Read the model definition and answer for the solid it produces. Units are mm, in the model's axes. Give positions to 0.01 mm unless a question says otherwise; leave off trailing zeros. Order: outer loops, then holes, each group sorted by start corner. A loop starts at its lowest first (then second) coordinate and runs counter-clockwise, first axis right, second up. Notation, with made-up numbers: (-6.5, 82) - (29.5, 82) arc R14 ccw to (29.5, 100) - close; hole circle Ø8 at (69, 58). An arc over 180 degrees is marked (long way). Answer as CSV lines item,"result". Start each with the question number.
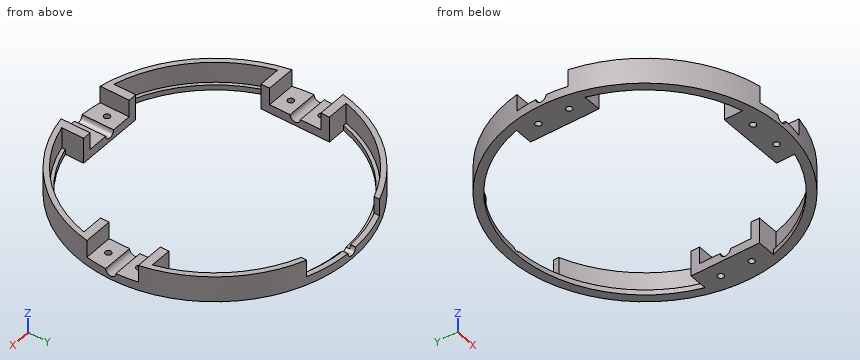
Autodesk Fusion 360 part; units mm, degrees
sketch "Sketch1" plane through (0, 0, 0) normal (0, 0, 1) x (1, 0, 0)
  circle A0 centre (0, 0) radius 80
  circle A1 centre (0, 0) radius 75
  line L0 (109.3577, 15) -> (-93.0881, 15) construction
  line L1 (20, 0) -> (2.5, 0)
  line L2 (109.3577, -15) -> (-93.0881, -15) construction
  line L3 (-78.5812, 15) -> (-61.5812, 15)
  line L4 (-78.5812, -15) -> (-61.5812, -15)
  line L5 (-97.5254, 20) -> (90.0497, 20) construction
  line L6 (-97.5254, -20) -> (90.0497, -20) construction
  line L7 (-77.4597, 20) -> (-61.5812, 20)
  line L8 (-77.4597, -20) -> (-61.5812, -20)
  line L9 (-61.5812, -15) -> (-61.5812, -20)
  line L10 (-61.5812, 15) -> (-61.5812, 20)
  line L11 (-20, -77.4597) -> (-20, -61.5812)
  line L12 (-15, -61.5812) -> (-20, -61.5812)
  line L13 (-15, -78.5812) -> (-15, -61.5812)
  line L14 (15, -78.5812) -> (15, -61.5812)
  line L15 (15, -61.5812) -> (20, -61.5812)
  line L16 (20, -77.4597) -> (20, -61.5812)
  line L17 (77.4597, -20) -> (61.5812, -20)
  line L18 (61.5812, -15) -> (61.5812, -20)
  line L19 (78.5812, -15) -> (61.5812, -15)
  line L20 (78.5812, 15) -> (61.5812, 15)
  line L21 (61.5812, 15) -> (61.5812, 20)
  line L22 (77.4597, 20) -> (61.5812, 20)
  line L23 (-28, 82.3691) -> (-28, 36.8916) construction
  line L24 (0, 2.5) -> (0, 20)
  line L25 (28, 82.3691) -> (28, 36.8916) construction
  line L26 (-33, 78.0405) -> (-33, 48.5416) construction
  line L27 (33, 78.0405) -> (33, 48.5416) construction
  line L28 (-28, 74.94) -> (-28, 69.5773)
  line L29 (28, 74.94) -> (28, 69.5773)
  line L30 (-61.5812, 15) -> (-61.5812, -15)
  line L31 (-15, -61.5812) -> (15, -61.5812)
  line L32 (61.5812, -15) -> (61.5812, 15)
  circle A2 centre (0, 0) radius 77
  dimension "d1" = 160
  dimension "d2" = -5
  dimension "d3" = 15
  dimension "d4" = 17
  dimension "d5" = 17
  dimension "d6" = 20
  dimension "d8" = 360
  dimension "d9" = 28
  dimension "d10" = 33
  dimension "d13" = -3
extrude "Extrude1" add sketch "Sketch1" along normal blind 15 contours A0 L20 L22 A2 | A0 L17 L19 A2 | A0 L22 L29 A2 | A1 L20 L22 A2 | A0 L16 L17 A2 | A1 L17 L19 A2 | A0 L28 L29 A2 | A1 L22 L29 A2 | A1 L20 L21 L22 | A0 L14 L16 A2 | A1 L16 L17 A2 | A1 L17 L18 L19 | A0 L7 L28 A2 | A1 L28 L29 A2 | A1 L14 L16 A2 | A0 L3 L7 A2 | A1 L7 L28 A2 | A0 L11 L13 A2 | A1 L14 L15 L16 | A1 L3 L7 A2 | A0 L8 L11 A2 | A1 L11 L13 A2 | A0 L4 L8 A2 | A1 L3 L7 L10 | A1 L8 L11 A2 | A1 L11 L12 L13 | A1 L4 L8 A2 | A1 L4 L8 L9 makes body 1 at (-69.1013, 40.3114, 10) makes body 2 at (18.8878, -77.7383, 5) makes body 3 at (-77.7383, -18.8878, 5)
extrude "Extrude2" add sketch "Sketch1" along normal blind 5 contours A0 L19 L20 A2 | A0 L20 L22 A2 | A0 L17 L19 A2 | A1 L19 L20 A2 | A1 L20 L22 A2 | A1 L17 L19 A2 | A1 L20 L21 L22 | A1 L19 L20 L32 | A0 L14 L16 A2 | A1 L17 L18 L19 | A0 L13 L14 A2 | A1 L14 L16 A2 | A0 L3 L7 A2 | A0 L11 L13 A2 | A1 L13 L14 A2 | A1 L14 L15 L16 | A0 L3 L4 A2 | A1 L3 L7 A2 | A1 L11 L13 A2 | A1 L13 L14 L31 | A0 L4 L8 A2 | A1 L3 L4 A2 | A1 L3 L7 L10 | A1 L11 L12 L13 | A1 L4 L8 A2 | A1 L3 L4 L30 | A1 L4 L8 L9 bodies 1 2 3
sketch "Sketch2" plane through (0, 0, 15) normal (0, 0, 1) x (-1, 0, 0)
  arc A0 (78.5812, 15) -> (15, 78.5812) centre (0, 0) ccw
  line L0 (15, 78.5812) -> (15, 61.5812)
  line L1 (15, 61.5812) -> (20, 61.5812)
  line L2 (20, 61.5812) -> (20, 72.2842)
  arc A1 (72.2842, 20) -> (20, 72.2842) centre (0, 0) ccw
  line L3 (72.2842, 20) -> (61.5812, 20)
  line L4 (61.5812, 20) -> (61.5812, 15)
  line L5 (61.5812, 15) -> (78.5812, 15)
  circle A2 centre (0, 0) radius 80
  circle A3 centre (0, 0) radius 77
  circle A4 centre (0, 0) radius 75
  line L6 (97.5254, 20) -> (-90.0497, 20)
  line L7 (97.5254, -20) -> (-90.0497, -20)
  line L8 (-20, 77.4597) -> (-20, 61.5812)
  line L9 (20, 77.4597) -> (20, 61.5812)
  line L10 (20, 72.2842) -> (20, 77.4597)
  line L11 (-20, 72.2842) -> (-20, 77.4597)
  line L12 (-72.2842, 20) -> (-77.4597, 20)
  line L13 (-72.2842, -20) -> (-77.4597, -20)
  line L14 (77.4597, 20) -> (72.2842, 20)
  line L15 (77.4597, -20) -> (72.2842, -20)
  dimension "d16" = -3
  dimension "d17" = -5
  dimension "d18" = 160
extrude "Extrude3" cut sketch "Sketch2" against normal blind 12 contours A1 A3 A4 L6 L9 L10 L14 | A3 A4 L7 L13 L15 | A3 A4 L6 L8 L11 L12 bodies 1
sketch "Sketch3" plane through (0, 0, 0) normal (0, 0, -1) x (1, 0, 0)
  arc A0 (-20, 72.2842) -> (-72.2842, 20) centre (0, 0) ccw
  line L0 (-20, 72.2842) -> (-20, 61.5812)
  line L1 (-20, 61.5812) -> (20, 61.5812)
  line L2 (20, 61.5812) -> (20, 72.2842)
  arc A1 (72.2842, 20) -> (20, 72.2842) centre (0, 0) ccw
  line L3 (72.2842, 20) -> (61.5812, 20)
  line L4 (61.5812, 20) -> (61.5812, -20)
  line L5 (61.5812, -20) -> (72.2842, -20)
  arc A2 (-72.2842, -20) -> (72.2842, -20) centre (0, 0) ccw
  line L6 (-72.2842, -20) -> (-61.5812, -20)
  line L7 (-61.5812, -20) -> (-61.5812, 20)
  line L8 (-61.5812, 20) -> (-72.2842, 20)
  circle A3 centre (0, 0) radius 70 construction
  line L9 (-17, 70) -> (15.5974, 70) construction
  circle A4 centre (9, 70) radius 1.75
  circle A5 centre (-9, 70) radius 1.75
  circle A6 centre (-70, 9) radius 1.75
  circle A7 centre (-70, -9) radius 1.75
  circle A8 centre (70, -9) radius 1.75
  circle A9 centre (70, 9) radius 1.75
  circle A10 centre (0, 0) radius 80
  dimension "d21" = 140
  dimension "d22" = 3.5
  dimension "d23" = 3.5
  dimension "d24" = 9
  dimension "d25" = 9
  dimension "d27" = 360
extrude "Extrude4" cut sketch "Sketch3" against normal blind 5 contours A4 | A5 | A6 | A7 | A8 | A9 bodies 1
sketch "Sketch4" plane through (0, 0, 15) normal (0, 0, 1) x (-1, 0, 0)
  line L0 (61.5812, -20) -> (74.3572, -20)
  arc A0 (-74.3572, -20) -> (74.3572, -20) centre (0, 0) ccw
  line L1 (-74.3572, -20) -> (-61.5812, -20)
  line L2 (-61.5812, -20) -> (-61.5812, -15)
  line L3 (-61.5812, -15) -> (-78.5812, -15)
  arc A1 (-78.5812, -15) -> (78.5812, -15) centre (0, 0) ccw
  line L4 (78.5812, -15) -> (61.5812, -15)
  line L5 (61.5812, -15) -> (61.5812, -20)
  line L6 (28, -82.3691) -> (28, -36.8916)
  line L7 (-28, -82.3691) -> (-28, -36.8916)
  circle A2 centre (0, 0) radius 75
  circle A3 centre (0, 0) radius 80
  line L8 (28, -74.94) -> (28, -69.5773)
  line L9 (-28, -74.94) -> (-28, -69.5773)
extrude "Extrude5" cut sketch "Sketch4" against normal blind 10 contours A0 L6 L7 A2 L8 L9 | A0 A1 L6 L7 A3 L8 L9 bodies 1
sketch "Sketch5" plane through (0, -61.5812, 0) normal (0, 1, 0) x (-1, 0, 0)
  line L0 (-15, 5) -> (-15, 15)
  line L1 (-15, 15) -> (-20, 15)
  line L2 (-20, 15) -> (-20, 0)
  line L3 (-20, 0) -> (20, 0)
  line L4 (20, 0) -> (20, 15)
  line L5 (20, 15) -> (15, 15)
  line L6 (15, 15) -> (15, 5)
  line L7 (15, 5) -> (-15, 5)
  circle A0 centre (0, 5) radius 3
  dimension "d32" = 6
extrude "Extrude6" cut sketch "Sketch5" against normal blind 18.419 contours L7 A0 picked at (-0.7219, 4.1708) bodies 1
pattern_circular "C-Pattern1" count 4 over 360 about axis through (0, 0, 1.75) along (0, 0, 1) of "Extrude6"
(1) Section B-B, the plane x = -42 is taken. Write down the section's boundary in (y, z), and give its area (3 significant figures).
(2) Section C-C, the plane z = 12 is taken. Write down the section's boundary in (x, y), and give its area (3 significant figures).
(3) Flat-ended cylindrical pins translate along their axes: pin 1 Ø4.5 at (x, y) = (70, 9) entering from +Z; pin 2 Ø5 at (y, z) = (30, 8.5) entering from -X; pin 3 Ø4 at (x, z) = (-70, 8.5) entering from -Y. Find the tip coordinate at first contact, or state that the pin passes through.
(4) Straight lines are drawn through the part: line 1 (X direction, y = -9, z = 3.25); line 2 (Y direction, x = -70, z = 3.5); line 3 (Y direction, x = -3, z = 0.75). For each, find the intervals that lie inside material, in ascending order. Write a range as [from, to].
(5) Section A-A, the plane y = 56 is taken. Write down the section's boundary in (x, z).
Checks:
1,outline,"(-68.09, 0) - (-62.14, 0) - (-62.14, 3) - (-64.54, 3) - (-64.54, 15) - (-68.09, 15) - close; (62.14, 0) - (68.09, 0) - (68.09, 15) - (64.54, 15) - (64.54, 3) - (62.14, 3) - close"
1,area,"121 mm²"
2,outline,"(-78.58, -15) arc R80 ccw to (-15, -78.58) - (-15, -61.58) - (-20, -61.58) - (-20, -74.36) arc R77 cw to (-74.36, -20) - (-61.58, -20) - (-61.58, -15) - close; (-78.58, 15) - (-61.58, 15) - (-61.58, 20) - (-74.36, 20) arc R77 cw to (-28, 71.73) - (-28, 74.94) arc R80 ccw to start; (15, -78.58) arc R80 ccw to (78.58, -15) - (61.58, -15) - (61.58, -20) - (74.36, -20) arc R77 cw to (20, -74.36) - (20, -61.58) - (15, -61.58) - close; (28, 71.73) arc R77 cw to (74.36, 20) - (61.58, 20) - (61.58, 15) - (78.58, 15) arc R80 ccw to (28, 74.94) - close"
2,area,"1,440 mm²"
3,pin 1,"stops at z = 5"
3,pin 2,"stops at x = -75.12"
3,pin 3,"stops at y = -42.14"
4,line 1,"x = [-79.49, -71.75], [-68.25, -61.58], [61.58, 68.25], [71.75, 79.49]"
4,line 2,"y = [-38.73, -32.08], [-20, -10.75], [-7.25, -2.6], [2.6, 7.25], [10.75, 20], [32.08, 38.73]"
4,line 3,"y = [-79.94, -61.58], [74.94, 79.94]"
5,outline,"(-57.13, 0) - (-49.89, 0) - (-49.89, 3) - (-52.85, 3) - (-52.85, 15) - (-57.13, 15) - close; (49.89, 0) - (57.13, 0) - (57.13, 15) - (52.85, 15) - (52.85, 3) - (49.89, 3) - close"
